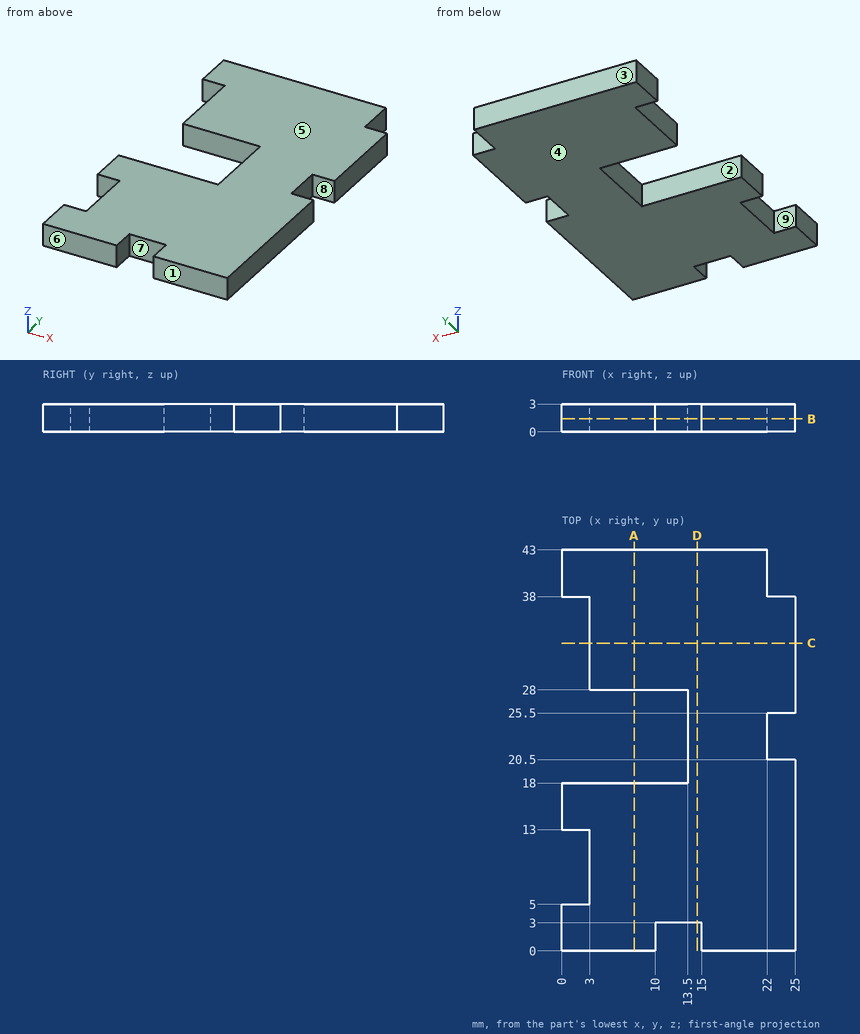
The figure shows three views and two pictorial views of one solid part (mm, origin at its lowest corner). Answer the questions. A direction names the side the tool comes from. Give positions to 0.01 mm unless a question says otherwise; leave off trailing zeros. Loops run counter-clockwise (first coordinate to the right, second up) from the corner with the lowest first, then second, coordinate; pieces in that order, holes last. Notation, with made-up numbers: (25, 17.25) -> (65, 17.25) arc R34 cw to (65, 52.25) -> close; hole circle Ø3 at (56.25, 74.5). An arc over 180 degrees is marked (long way). Put each result on its own line as item: value. Start each with the question number.
Item 1: The part is cut by section C-C (y = 33). Give the vertices of the cut face in (x, z), then the cut area to 3 significant figures.
Item 2: Each of these flat-tipped pins is pushed along its axis until it touches: P1, Ø1.5, axis at y = 10.5, z = 1, coming from the -X side; P2, Ø1.5, axis at x = 13, z = 2, coming from the -Y side; P3, Ø1.5, axis at y = 23.5, z = 1.5, coming from the +X side; P4, Ø1.5, axis at y = 1, z = 1, coming from the -X side. Where does it stop, or does it pass through?
Item 3: Which of the six approach directions +Z, -Z, +X, -X, +Y, -Y give full straight-line access (tool end or side, diameter ignored) to the marked faces 5, 6, 7, 8 and 9?
Item 4: The mould has two halves that part along Y. Classify the marked faces 1, 2, 3 and 4: released by +Y, released by -Y, zero draft, split by the parting line, or undercut.
Item 5: The part is cut by section D-D (x = 14.5). Give the vertices of the cut face in (y, z), then the cut area to 3 significant figures.
Item 6: The part is cut by section B-B (z = 1.4). Give the vertices of the cut face in (x, y), then the cut area to 3 significant figures.
Item 7: Find the intervals of material crossed by L1, parallel to Y at x = 11.25, z = 0.6; L2, parallel to Y at x = 9, z = 1.65; L3, parallel to X at y = 10.5, z = 2.6, in increasing order. Write a range as [from, to].
Item 8: The part is cut by section A-A (x = 7.75). Give the vertices of the cut face in (y, z).
Answers below:
1. outline: (3, 0) -> (25, 0) -> (25, 3) -> (3, 3) -> close
1. area: 66.0 mm2
2. P1: x = 3
2. P2: y = 3
2. P3: x = 22
2. P4: x = 0
3. face 5: +Z, +X, -X, +Y, -Y
3. face 6: +Z, -Z, +X, -X, -Y
3. face 7: +Z, -Z, -Y
3. face 8: +Z, -Z, +X
3. face 9: +Z, -Z, -X
4. face 1: released by -Y
4. face 2: undercut
4. face 3: released by +Y
4. face 4: zero draft
5. outline: (3, 0) -> (43, 0) -> (43, 3) -> (3, 3) -> close
5. area: 120 mm2
6. outline: (0, 0) -> (10, 0) -> (10, 3) -> (15, 3) -> (15, 0) -> (25, 0) -> (25, 20.5) -> (22, 20.5) -> (22, 25.5) -> (25, 25.5) -> (25, 38) -> (22, 38) -> (22, 43) -> (0, 43) -> (0, 38) -> (3, 38) -> (3, 28) -> (13.5, 28) -> (13.5, 18) -> (0, 18) -> (0, 13) -> (3, 13) -> (3, 5) -> (0, 5) -> close
6. area: 841 mm2
7. L1: [3, 18], [28, 43]
7. L2: [0, 18], [28, 43]
7. L3: [3, 25]
8. outline: (0, 0) -> (18, 0) -> (18, 3) -> (0, 3) -> close; (28, 0) -> (43, 0) -> (43, 3) -> (28, 3) -> close
